Part model, mm, in its own coordinate system. Round coordinates to 2 decimals unless told otherwise and drop trailing zeros. Loops run counter-clockwise (first coordinate to the right, second up) from the corner with the lowest first, then second, coordinate; pieces in that order, holes last. Notation, with made-up numbers: M 73.5,-31 L 78.5,-31 A6 cw 78.5,-25 Z; hole C 58.25,-7 d7. An arc over 180 degrees is marked long. Answer as CSV lines item,"result". Start each with the question number.
Item 1: Drop a flat-ended pin along its axis: pin 1 Ø2 at (x, y) = (92, -42) entering from -Z. Give the stop position or say it passes through.
Item 2: Wall check: line 1 (Y direction, x = 92, z = 2.3); line 2 (X direction, y = 41.5, z = 2.3). Give the ranges that are in metal, low to high.
Item 3: Band-saw the part on B-B (x = 92). Give the cut face in (y, z).
Item 4: Mould opens along X. For faces 1 (the flat face through (51, -51.5, 1)), 2 (the cylindrical face through (6.75, 41.95, 1.48)), 3 (the flat face through (-1.5, -1, 1)) say: pulls with the +X half, pulls with the -X half, needs draft (parallel to the pull), parting line crosses it, or undercut.
Item 5: Band-saw the part on A-A (y = -42). Give the cut face in (x, z).
Autodesk Inventor part; units mm, degrees
ref_plane "YZ Plane" through (0, 0, 0) normal (1, 0, 0) x (0, 1, 0)
ref_plane "XZ Plane" through (0, 0, 0) normal (0, 1, 0) x (-1, 0, 0)
ref_plane "XY Plane" through (0, 0, 0) normal (0, 0, 1) x (1, 0, 0)
sketch "Boceto1" plane through (0, 0, 0) normal (0, 0, 1) x (1, 0, 0)
  line L0 (-1.5, -51.5) -> (-1.5, 51.5)
  line L1 (98.5, -51.5) -> (18.2, -51.5)
  line L2 (101.5, 51.5) -> (101.5, -51.5)
  line L3 (101.5, -51.5) -> (-1.5, -51.5)
  line L4 (-1.5, -51.5) -> (-1.5, 51.5)
  line L5 (-1.5, 51.5) -> (101.5, 51.5)
  line L6 (101.5, 51.5) -> (101.5, -51.5)
  circle A0 centre (8, -42) radius 1.25
  circle A1 centre (8, 42) radius 1.25
  circle A2 centre (92, 42) radius 1.25
  circle A3 centre (92, -42) radius 1.25
  point P0 (0, 0)
extrude "Extrusión1" add sketch "Boceto1" along normal blind 3
properties part number "Tapa_abajo"
Answer block:
1,pin 1,"passes through"
2,line 1,"y = -51.5 to -43.25, -40.75 to 40.75, 43.25 to 51.5"
2,line 2,"x = -1.5 to 6.85, 9.15 to 90.85, 93.15 to 101.5"
3,outline,"M -51.5,0 L -43.25,0 L -43.25,3 L -51.5,3 Z; M -40.75,0 L 40.75,0 L 40.75,3 L -40.75,3 Z; M 43.25,0 L 51.5,0 L 51.5,3 L 43.25,3 Z"
4,face 1,"needs draft"
4,face 2,"undercut"
4,face 3,"pulls with the -X half"
5,outline,"M -1.5,0 L 6.75,0 L 6.75,3 L -1.5,3 Z; M 9.25,0 L 90.75,0 L 90.75,3 L 9.25,3 Z; M 93.25,0 L 101.5,0 L 101.5,3 L 93.25,3 Z"
